Verification items for the finished model (mm, model axes). Coordinates: 2 decimals unless noted, no trailing zeros. Write each loop counter-clockwise with the first axis right and the second up, starting at its lowest first coordinate (ties: lowest second). Pieces come first, ordered by that corner, then holes. Notation, with made-up numbers: (-36, 45.25) - (-27, 45.25) arc R17 ccw to (-27, 61.25) - close; hole circle Ø9 at (78, 38). An arc over 180 degrees is marked (long way). Use one line per item in the form item = value. Start each with the question number.
(1) Sectioned sample at C-C (y = 22). Record the cut outline in (x, z).
(2) Sectioned sample at A-A (x = 0). Record the cut outline in (y, z) (3 decimals).
(3) Material ranges on line 1 (Y direction, x = 22.5, z = 3.1); line 2 (Y direction, x = 1, z = 0.75); line 3 (X direction, y = -25.5, z = 4.95), recorded low to high. Write a range as [from, to].
(4) Sectioned sample at B-B (y = -16.75). Record the cut outline in (x, z), and give its area (3 significant figures).
(5) Sectioned sample at D-D (z = 5). Count the separate pieces of the cut face and the enclosed holes in it, and give its area (3 significant figures).
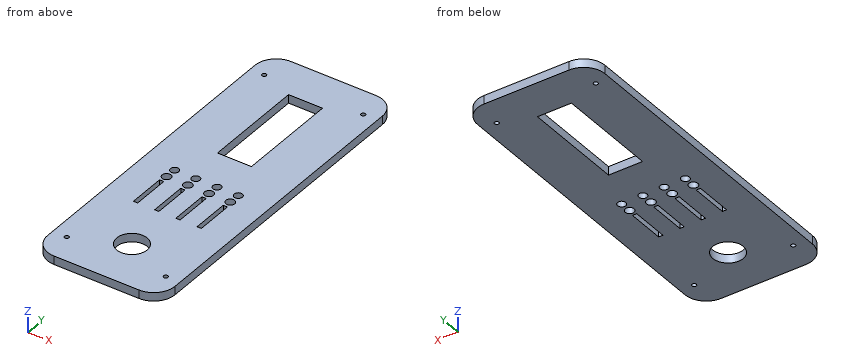
from build123d import *

# Parameters (mm, degrees)
F1_DEPTH = 6
F2_W     = 24
F2_H     = 72
F3_DEPTH = 6
F4_W     = 3
F4_H     = 26.5
F4_R     = 2.9
F4_R_2   = 3.15
F5_DEPTH = 6
F6_R     = 10.75
F7_DEPTH = 6
F8_R     = 1.5
F9_DEPTH = 6


with BuildPart() as f1:
    # F0 (on Top) → F1 (new body)
    with BuildSketch(Plane.XY):
        with BuildLine():
            Line((-30, -120), (30, -120))
            ThreePointArc((30, -120), (40.606602, -115.606602), (45, -105))
            Line((45, -105), (45, 105))
            ThreePointArc((45, 105), (40.606602, 115.606602), (30, 120))
            Line((30, 120), (-30, 120))
            ThreePointArc((-30, 120), (-40.606602, 115.606602), (-45, 105))
            Line((-45, 105), (-45, -105))
            ThreePointArc((-45, -105), (-40.606602, -115.606602), (-30, -120))
        make_face()
    extrude(amount=F1_DEPTH)

    # F2 (on face) → F3 (cut, through all)
    with BuildSketch(Plane.XY.offset(6)):
        with Locations((0, 55.712325)):
            Rectangle(F2_W, F2_H)
    extrude(amount=-F3_DEPTH, mode=Mode.SUBTRACT)

    # F4 (on face) → F5 (cut, through all)
    with BuildSketch(Plane.XY.offset(6)):
        with Locations((-22.5, -35)):
            Rectangle(F4_W, F4_H)
        with Locations((-22.433495, -8.750276)):
            Circle(F4_R)
        with Locations((-22.5, -16.75)):
            Circle(F4_R_2)
        with Locations((-7.5, -16.75)):
            Circle(F4_R_2)
        with Locations((-7.5, -35)):
            Rectangle(F4_W, F4_H)
        with Locations((-7.433495, -8.750276)):
            Circle(F4_R)
        with Locations((7.5, -16.75)):
            Circle(F4_R_2)
        with Locations((7.5, -35)):
            Rectangle(F4_W, F4_H)
        with Locations((7.566505, -8.750276)):
            Circle(F4_R)
        with Locations((22.5, -16.75)):
            Circle(F4_R_2)
        with Locations((22.5, -35)):
            Rectangle(F4_W, F4_H)
        with Locations((22.566505, -8.750276)):
            Circle(F4_R)
    extrude(amount=-F5_DEPTH, mode=Mode.SUBTRACT)

    # F6 (on face) → F7 (cut, through all)
    with BuildSketch(Plane.XY.offset(6)):
        with Locations((0, -84.125)):
            Circle(F6_R)
    extrude(amount=-F7_DEPTH, mode=Mode.SUBTRACT)

    # F8 (on face) → F9 (cut, through all)
    with BuildSketch(Plane.XY.offset(6)):
        with Locations((-35, -100)):
            Circle(F8_R)
        with Locations((35, -100)):
            Circle(F8_R)
        with Locations((35, 100)):
            Circle(F8_R)
        with Locations((-35, 100)):
            Circle(F8_R)
    extrude(amount=-F9_DEPTH, mode=Mode.SUBTRACT)


solid = f1.part
Answers below:
q1.outline = (-45, 0) - (-12, 0) - (-12, 6) - (-45, 6) - close; (12, 0) - (45, 0) - (45, 6) - (12, 6) - close
q2.outline = (-120, 0) - (-94.875, 0) - (-94.875, 6) - (-120, 6) - close; (-73.375, 0) - (19.712, 0) - (19.712, 6) - (-73.375, 6) - close; (91.712, 0) - (120, 0) - (120, 6) - (91.712, 6) - close
q3.line_1 = [-120, -48.25], [-21.75, -19.9], [-13.6, -11.65], [-5.85, 120]
q3.line_2 = [-120, -94.83], [-73.42, 19.71], [91.71, 120]
q3.line_3 = [-45, -24], [-21, -9], [-6, 6], [9, 21], [24, 45]
q4.outline = (-45, 0) - (-25.65, 0) - (-25.65, 6) - (-45, 6) - close; (-19.35, 0) - (-10.65, 0) - (-10.65, 6) - (-19.35, 6) - close; (-4.35, 0) - (4.35, 0) - (4.35, 6) - (-4.35, 6) - close; (10.65, 0) - (19.35, 0) - (19.35, 6) - (10.65, 6) - close; (25.65, 0) - (45, 0) - (45, 6) - (25.65, 6) - close
q4.area = 389 mm2
q5.separate_pieces = 1
q5.enclosed_holes = 18
q5.area = 18,700 mm2
